Read the model definition and answer for the solid it produces. Units are mm, in the model's axes. Round coordinates to 2 decimals unless told otherwise and drop trailing zeros. One line per item, written item: value. Start each with the question number.
1. Consider line 1 (X direction, y = 1, z = 258); line 2 (X direction, y = 31.5, z = 504); line 3 (X direction, y = 17.5, z = 413.5). Determine where each line is inside the solid, lowest interval first.
2. Flat-ended cylindrical pins translate along their axes: pin 1 Ø5.5 at (x, z) = (-29.5, 747.5) entering from +Y; pin 2 Ø2.5 at (y, z) = (15.5, 718.5) entering from +X; pin 3 Ø1.5 at (y, z) = (16, 721.5) entering from -X. Find the tip coordinate at first contact, or state that the pin passes through.
3. Section A-A (z = 560) is taken. State how many separate pieces and enclosed holes the cut face has, then the cut area to 3 significant figures.
from build123d import *

# Parameters (mm, degrees)
F0_R     = 3.4
F1_DEPTH = 1060


# Not quite as in the source:
# - ends of sketch curves that miss each other by under 0.0002 mm in the source are joined


with BuildPart() as f1:
    # F0 (on Top) → F1 (new body)
    with BuildSketch(Plane.XY):
        with BuildLine():
            ThreePointArc((-37.8290628647, 13.3437199509), (-39.194573333, 10.8017277117), (-41.229063, 8.755464))
            ThreePointArc((-41.229063, 8.755464), (-43.8470969887, 8.5193960225), (-45.229063, 10.755464))
            Line((-45.229063, 10.755464), (-45.229063, 12.055464))
            ThreePointArc((-45.229063, 12.055464), (-45.3755096094, 12.4090173906), (-45.729063, 12.555464))
            Line((-45.729063, 12.555464), (-47.229063, 12.555464))
            ThreePointArc((-47.229063, 12.555464), (-48.996829953, 11.823230953), (-49.729063, 10.055464))
            Line((-49.729063, 10.055464), (-49.729063, -0.744536))
            ThreePointArc((-49.729063, -0.744536), (-48.996829953, -2.512302953), (-47.229063, -3.244536))
            Line((-47.229063, -3.244536), (-36.429063, -3.244536))
            ThreePointArc((-36.429063, -3.244536), (-34.661296047, -2.512302953), (-33.929063, -0.744536))
            Line((-33.929063, -0.744536), (-33.929063, 0.755464))
            ThreePointArc((-33.929063, 0.755464), (-34.0755096094, 1.1090173906), (-34.429063, 1.255464))
            Line((-34.429063, 1.255464), (-35.729063, 1.255464))
            ThreePointArc((-35.729063, 1.255464), (-37.9651309775, 2.6374300113), (-37.729063, 5.255464))
            ThreePointArc((-37.729063, 5.255464), (-35.6827992883, 7.289953667), (-33.1408070491, 8.6554641353))
            ThreePointArc((-33.1408070491, 8.6554641353), (-32.7208836531, 8.767678459), (-32.287871, 8.805464))
            Line((-32.287871, 8.805464), (-27.170255, 8.805464))
            ThreePointArc((-27.170255, 8.805464), (-26.7372423469, 8.767678459), (-26.3173189877, 8.6554640338))
            ThreePointArc((-26.3173189877, 8.6554640338), (-23.7753267117, 7.289953667), (-21.729063, 5.255464))
            ThreePointArc((-21.729063, 5.255464), (-21.4929950225, 2.6374300113), (-23.729063, 1.255464))
            Line((-23.729063, 1.255464), (-25.029063, 1.255464))
            ThreePointArc((-25.029063, 1.255464), (-25.3826163906, 1.1090173906), (-25.529063, 0.755464))
            Line((-25.529063, 0.755464), (-25.529063, -0.744536))
            ThreePointArc((-25.529063, -0.744536), (-24.796829953, -2.512302953), (-23.029063, -3.244536))
            Line((-23.029063, -3.244536), (-12.229063, -3.244536))
            ThreePointArc((-12.229063, -3.244536), (-10.461296047, -2.512302953), (-9.729063, -0.744536))
            Line((-9.729063, -0.744536), (-9.729063, 10.055464))
            ThreePointArc((-9.729063, 10.055464), (-10.461296047, 11.823230953), (-12.229063, 12.555464))
            Line((-12.229063, 12.555464), (-13.729063, 12.555464))
            ThreePointArc((-13.729063, 12.555464), (-14.0826163906, 12.4090173906), (-14.229063, 12.055464))
            Line((-14.229063, 12.055464), (-14.229063, 10.755464))
            ThreePointArc((-14.229063, 10.755464), (-15.6110290113, 8.5193960225), (-18.229063, 8.755464))
            ThreePointArc((-18.229063, 8.755464), (-20.263552667, 10.8017277117), (-21.6290631353, 13.3437199509))
            ThreePointArc((-21.6290631353, 13.3437199509), (-21.741277459, 13.7636433469), (-21.779063, 14.196656))
            Line((-21.779063, 14.196656), (-21.779063, 19.314273))
            ThreePointArc((-21.779063, 19.314273), (-21.741277459, 19.7472856531), (-21.6290630338, 20.1672090123))
            ThreePointArc((-21.6290630338, 20.1672090123), (-20.2635523872, 22.7092006659), (-18.229063, 24.755464))
            ThreePointArc((-18.229063, 24.755464), (-15.6110290113, 24.9915319775), (-14.229063, 22.755464))
            Line((-14.229063, 22.755464), (-14.229063, 21.455464))
            ThreePointArc((-14.229063, 21.455464), (-14.0826163906, 21.1019106094), (-13.729063, 20.955464))
            Line((-13.729063, 20.955464), (-12.229063, 20.955464))
            ThreePointArc((-12.229063, 20.955464), (-10.461296047, 21.687697047), (-9.729063, 23.455464))
            Line((-9.729063, 23.455464), (-9.729063, 34.255464))
            ThreePointArc((-9.729063, 34.255464), (-10.461296047, 36.023230953), (-12.229063, 36.755464))
            Line((-12.229063, 36.755464), (-23.029063, 36.755464))
            ThreePointArc((-23.029063, 36.755464), (-24.796829953, 36.023230953), (-25.529063, 34.255464))
            Line((-25.529063, 34.255464), (-25.529063, 32.755464))
            ThreePointArc((-25.529063, 32.755464), (-25.3826163906, 32.4019106094), (-25.029063, 32.255464))
            Line((-25.029063, 32.255464), (-23.729063, 32.255464))
            ThreePointArc((-23.729063, 32.255464), (-21.4929950225, 30.8734979887), (-21.729063, 28.255464))
            ThreePointArc((-21.729063, 28.255464), (-23.7753267117, 26.220974333), (-26.3173189509, 24.8554638647))
            ThreePointArc((-26.3173189509, 24.8554638647), (-26.7372423469, 24.743249541), (-27.170255, 24.705464))
            Line((-27.170255, 24.705464), (-32.287871, 24.705464))
            ThreePointArc((-32.287871, 24.705464), (-32.7208836531, 24.743249541), (-33.1408070123, 24.8554639662))
            ThreePointArc((-33.1408070123, 24.8554639662), (-35.6827992883, 26.220974333), (-37.729063, 28.255464))
            ThreePointArc((-37.729063, 28.255464), (-37.9651309775, 30.8734979887), (-35.729063, 32.255464))
            Line((-35.729063, 32.255464), (-34.429063, 32.255464))
            ThreePointArc((-34.429063, 32.255464), (-34.0755096094, 32.4019106094), (-33.929063, 32.755464))
            Line((-33.929063, 32.755464), (-33.929063, 34.255464))
            ThreePointArc((-33.929063, 34.255464), (-34.661296047, 36.023230953), (-36.429063, 36.755464))
            Line((-36.429063, 36.755464), (-47.229063, 36.755464))
            ThreePointArc((-47.229063, 36.755464), (-48.996829953, 36.023230953), (-49.729063, 34.255464))
            Line((-49.729063, 34.255464), (-49.729063, 23.455464))
            ThreePointArc((-49.729063, 23.455464), (-48.996829953, 21.687697047), (-47.229063, 20.955464))
            Line((-47.229063, 20.955464), (-45.729063, 20.955464))
            ThreePointArc((-45.729063, 20.955464), (-45.3755096094, 21.1019106094), (-45.229063, 21.455464))
            Line((-45.229063, 21.455464), (-45.229063, 22.755464))
            ThreePointArc((-45.229063, 22.755464), (-43.8470969887, 24.9915319775), (-41.229063, 24.755464))
            ThreePointArc((-41.229063, 24.755464), (-39.1945736128, 22.7092006659), (-37.8290631854, 20.1672089327))
            ThreePointArc((-37.8290631854, 20.1672089327), (-37.716848541, 19.7472856531), (-37.679063, 19.314273))
            Line((-37.679063, 19.314273), (-37.679063, 14.196656))
            ThreePointArc((-37.679063, 14.196656), (-37.716848541, 13.7636433469), (-37.8290628647, 13.3437199509))
        make_face()
        Polygon((-43.257983, -0.764408), (-45.929556, -0.764408), (-46.636663, -1.471515), (-48.050877, -0.057301), (-47.34377, 0.649805), (-47.34377, 3.321378), (-48.050877, 4.028485), (-46.636663, 5.442699), (-45.929556, 4.735592), (-43.257983, 4.735592), (-42.550877, 5.442699), (-41.136663, 4.028485), (-41.84377, 3.321378), (-41.84377, 0.649805), (-41.136663, -0.057301), (-42.550877, -1.471515), align=None, mode=Mode.SUBTRACT)
        Polygon((-12.20919, 3.226544), (-12.20919, 0.554971), (-11.502084, -0.152136), (-12.916297, -1.566349), (-13.623404, -0.859242), (-16.294977, -0.859242), (-17.002084, -1.566349), (-18.416297, -0.152136), (-17.70919, 0.554971), (-17.70919, 3.226544), (-18.416297, 3.933651), (-17.002084, 5.347864), (-16.294977, 4.640758), (-13.623404, 4.640758), (-12.916297, 5.347864), (-11.502084, 3.933651), align=None, mode=Mode.SUBTRACT)
        with Locations((-29.729063, 16.755464)):
            Circle(F0_R, mode=Mode.SUBTRACT)
        Polygon((-47.248935, 30.284385), (-47.248935, 32.955957), (-47.956042, 33.663064), (-46.541829, 35.077278), (-45.834722, 34.370171), (-43.163149, 34.370171), (-42.456042, 35.077278), (-41.041829, 33.663064), (-41.748935, 32.955957), (-41.748935, 30.284385), (-41.041829, 29.577278), (-42.456042, 28.163064), (-43.163149, 28.870171), (-45.834722, 28.870171), (-46.541829, 28.163064), (-47.956042, 29.577278), align=None, mode=Mode.SUBTRACT)
        Polygon((-16.200143, 34.275337), (-13.52857, 34.275337), (-12.821463, 34.982444), (-11.407249, 33.56823), (-12.114356, 32.861123), (-12.114356, 30.18955), (-11.407249, 29.482444), (-12.821463, 28.06823), (-13.52857, 28.775337), (-16.200143, 28.775337), (-16.907249, 28.06823), (-18.321463, 29.482444), (-17.614356, 30.18955), (-17.614356, 32.861123), (-18.321463, 33.56823), (-16.907249, 34.982444), align=None, mode=Mode.SUBTRACT)
    extrude(amount=F1_DEPTH)


solid = f1.part
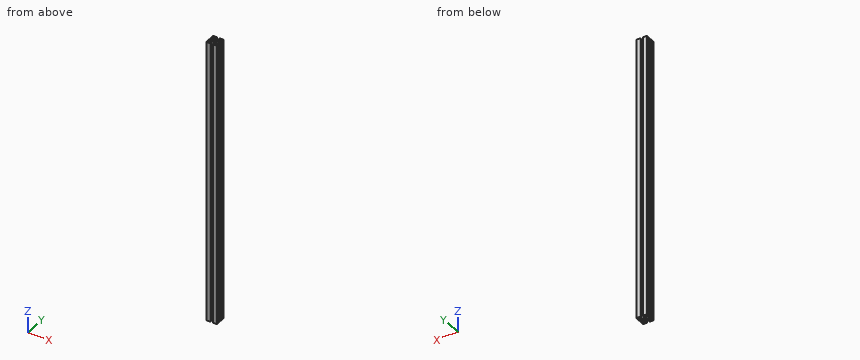
Answer:
1. line 1: -49.73 to -47.34, -41.84 to -33.99, -25.47 to -17.71, -12.21 to -9.73
1. line 2: -49.73 to -47.25, -41.75 to -37.52, -21.94 to -17.61, -12.11 to -9.73
1. line 3: -37.68 to -33.05, -26.41 to -21.78
2. pin 1: y = 24.74
2. pin 2: x = -21.78
2. pin 3: x = -37.68
3. separate pieces: 1
3. enclosed holes: 5
3. area: 828 mm^2
